The model under review builds one solid part; all positions refer to its coordinate system, in mm. Face numbers are marked on the shaded views. Coordinates: 2 decimals unless noted, no trailing zeros. Write each loop counter-clockwise with the first axis right and the second up, starting at its lowest first coordinate (ties: lowest second). Pieces come first, ordered by that corner, then holes. Notation, with made-up numbers: (-3.5, -34.75) - (33.5, -34.75) arc R33 ccw to (33.5, 1.25) - close; hole circle Ø9 at (81, 50.5). An arc over 180 degrees is marked (long way). Answer as CSV lines item,"result". Start each with the question number.
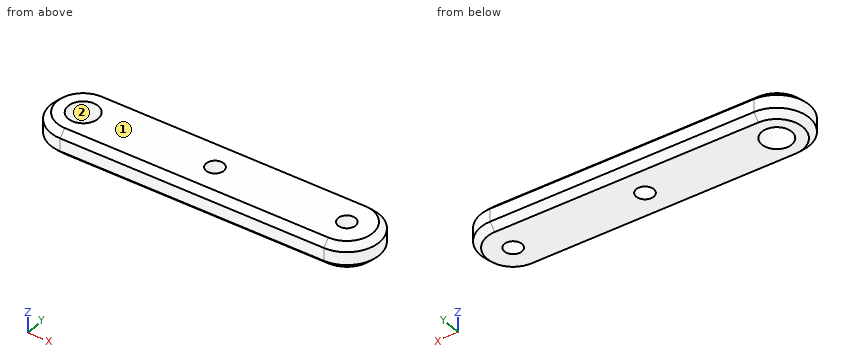
```python
from build123d import *

# Parameters (mm, degrees)
SKETCH1_R           = 1.35
SKETCH1_R_2         = 2.3
BOSS_EXTRUDE1_DEPTH = 4
CHAMFER1_SIZE       = 1


with BuildPart() as part:
    # Sketch1 → Boss-Extrude1 (new body)
    with BuildSketch(Plane.XY):
        with BuildLine():
            Line((40, 5), (0, 5))
            ThreePointArc((0, 5), (-5, 0), (0, -5))
            Line((0, -5), (40, -5))
            ThreePointArc((40, -5), (45, 0), (40, 5))
        make_face()
        with Locations((20, 0)):
            Circle(SKETCH1_R, mode=Mode.SUBTRACT)
        Circle(SKETCH1_R_2, mode=Mode.SUBTRACT)
        with Locations((40, 0)):
            Circle(SKETCH1_R, mode=Mode.SUBTRACT)
    extrude(amount=BOSS_EXTRUDE1_DEPTH)

    # Chamfer1
    chamfer1_edges = [part.edges().sort_by_distance(p)[0] for p in [
        (-5, 0, 0),
        (20, 5, 0),
        (45, 0, 0),
        (20, -5, 0),
        (45, 0, 4),
        (20, 5, 4),
        (-5, 0, 4),
        (20, -5, 4),
    ]]
    chamfer(chamfer1_edges, length=CHAMFER1_SIZE)


solid = part.part
```
(1) For pin 1 (3.5 mm diameter, centred on x = 40, y = 0, fed in from +Z), flat-tipped, find the tip position at first contact; note if it passes through.
(2) Wall thickness on line 1 (Y direction, x = 20, z = 2); line 2 (X direction, y = -0.25, z = 3.3); line 3 (X direction, y = -1, z = 1.65): over which ranges is each line inside the solid? List them lowest first.
(3) Add section B-B on z = 3.5. Give the boundary of the cut face in (x, y).
(4) The part is to be moulded in two halves that separate along X. For the marked faces 1 and 2, say which applies: released by +X, released by -X, zero draft, split by the parting line, or undercut.
(5) Add section D-D on x = 38. Give the boundary of the cut face in (y, z), then the cut area to 3 significant figures.
(6) Add section C-C on x = 20. Give the boundary of the cut face in (y, z), then the cut area to 3 significant figures.
(7) Add section A-A on y = 0. Give the boundary of the cut face in (x, z), then the cut area to 3 significant figures.
Reported:
1,pin 1,"z = 4"
2,line 1,"-5 to -1.35, 1.35 to 5"
2,line 2,"-4.69 to -2.29, 2.29 to 18.67, 21.33 to 38.67, 41.33 to 44.69"
2,line 3,"-4.9 to -2.07, 2.07 to 19.09, 20.91 to 39.09, 40.91 to 44.9"
3,outline,"(0, -4.5) - (40, -4.5) arc R4.5 ccw to (40, 4.5) - (0, 4.5) arc R4.5 ccw to start; hole circle Ø4.6 at (0, 0); hole circle Ø2.7 at (20, 0); hole circle Ø2.7 at (40, 0)"
4,face 1,"zero draft"
4,face 2,"undercut"
5,outline,"(-5, 1) - (-4, 0) - (4, 0) - (5, 1) - (5, 3) - (4, 4) - (-4, 4) - (-5, 3) - close"
5,area,"38.0 mm²"
6,outline,"(-5, 1) - (-4, 0) - (-1.35, 0) - (-1.35, 4) - (-4, 4) - (-5, 3) - close; (1.35, 0) - (4, 0) - (5, 1) - (5, 3) - (4, 4) - (1.35, 4) - close"
6,area,"27.2 mm²"
7,outline,"(-5, 1) - (-4, 0) - (-2.3, 0) - (-2.3, 4) - (-4, 4) - (-5, 3) - close; (2.3, 0) - (18.65, 0) - (18.65, 4) - (2.3, 4) - close; (21.35, 0) - (38.65, 0) - (38.65, 4) - (21.35, 4) - close; (41.35, 0) - (44, 0) - (45, 1) - (45, 3) - (44, 4) - (41.35, 4) - close"
7,area,"158 mm²"
